```python
from build123d import *

# Parameters (mm, degrees)
EXTRUDE_1_DEPTH     = 500
SKETCH_2_R          = 1.6
CUT_EXTRUDE_1_DEPTH = 1.15


with BuildPart() as part:
    # 草图1 → 凸台-拉伸1 (new body)
    with BuildSketch(Plane(origin=(0, 0, 0), x_dir=(1, 0, 0), z_dir=(0, 1, 0))):
        Polygon((0, -5), (8, -5), (8, 0), (5.75, 0), (5.75, -1.15), (6.85, -1.15), (6.85, -3.85), (1.15, -3.85), (1.15, -1.15), (2.25, -1.15), (2.25, 0), (0, 0), align=None)
    extrude(amount=EXTRUDE_1_DEPTH)

    # 草图2 → 切除-拉伸1 (cut)
    with BuildSketch(Plane.XY.offset(5)):
        with Locations((4, 80)):
            Circle(SKETCH_2_R)
    extrude(amount=-CUT_EXTRUDE_1_DEPTH, mode=Mode.SUBTRACT)


solid = part.part
```
Source: CAD feature listing. Evaluate the final solid. Frame: model axes, mm. Round coordinates to 2 decimals unless told otherwise and drop trailing zeros. Loops run counter-clockwise (first coordinate to the right, second up) from the corner with the lowest first, then second, coordinate; pieces in that order, holes last. Notation, with made-up numbers: M 84.25,74.5 L 89.25,74.5 A10 cw 89.25,91.5 Z; hole C 43,-4.75 d5. An arc over 180 degrees is marked long. Put each result on its own line as item: value.
(1) Ray query, line 1 (X direction, y = 80, z = 4.1); line 2 (Z direction, x = 6, y = 64); line 3 (X direction, y = 261, z = 3.55). Return the intervals inside material, ascending. Write a range as [from, to].
Solutions:
line 1: [0, 2.4], [5.6, 8]
line 2: [0, 1.15], [3.85, 5]
line 3: [0, 1.15], [6.85, 8]
(2) Section B-B, the plane y = 66.5. Return loops of the section in (x, z).
Solutions:
outline: M 0,0 L 2.25,0 L 2.25,1.15 L 1.15,1.15 L 1.15,3.85 L 6.85,3.85 L 6.85,1.15 L 5.75,1.15 L 5.75,0 L 8,0 L 8,5 L 0,5 Z
(3) First-contact query: pin 1 (1 mm diameter, centred on x = 3, z = 1, fed in from +Y). Flat tip, straight axial feed; report the tip coordinate or a pass-through.
Solutions:
pin 1: through
(4) Section A-A, the plane x = 4. Return loops of the section in (y, z).
Solutions:
outline: M 0,3.85 L 78.4,3.85 L 78.4,5 L 0,5 Z; M 81.6,3.85 L 500,3.85 L 500,5 L 81.6,5 Z
